Build history of the part. All positions in model axes, mm. A direction names the side the tool comes from. Give positions to 0.01 mm unless a question says otherwise; leave off trailing zeros. Write each loop counter-clockwise with the first axis right and the second up, starting at its lowest first coordinate (ties: lowest second). Pieces come first, ordered by that corner, then holes. Notation, with made-up numbers: (62.25, 54.25) -> (116.25, 54.25) arc R17 ccw to (116.25, 60.25) -> close; hole circle Ø8 at (-25.75, 75). An arc over 180 degrees is marked (long way). One line per question, with ' | ' between items. Start each with the question number.
(1) Tool access for faces 1 (the flat face through (24.25, -5, 59)), 2 (the cylindrical face through (-7.697, -19.028, 89.633)), 3 (the flat face through (8, 17, 91)): list every direction of +Z, -Z, +X, -X, +Y, -Y with a clear straight run to the whole face (end or side of a thin tool).
(2) Band-saw the part on C-C, the plane y = 9. Give the cut face in (x, z).
(3) Drill centre lines: probe 1 along X at (y, z) = (17.8, 91); probe 2 along X at (y, z) = (13.5, 66); probe 3 along Y at (x, z) = (3, 49). Where is each one in solid material? Low to high. Write a range as from..to.
(4) Band-saw the part on B-B, the plane x = -8. Give the cut face in (y, z).
(5) Band-saw the part on A-A, the plane z = 83.5. Give the cut face in (x, y).
(6) Pin check, flat tips, straight feed: P1, Ø8, axis at y = -7, z = 11, coming from the +X side; P2, Ø10, axis at x = 8.5, y = -1.5, coming from the +Z side; P3, Ø4, axis at x = 29, z = 11.5, coming from the -Y side. Stop position of each tip, or through.
(7) Band-saw the part on D-D, the plane z = 11. Give the cut face in (x, y).
(8) Pull direction Z, two halves, no side cores. Call faces 4 (the flat face through (3, 21, 46)), 5 (the flat face through (0, 0, 0)), 6 (the flat face through (23.25, 16, 21)): released by +Z, released by -Z, zero draft, split by the parting line, or undercut.
from build123d import *

# Parameters (mm, degrees)
SKETCH2_W                         = 48.5
SKETCH2_H                         = 42
SKETCH2_W_2                       = 38.5
SKETCH2_H_2                       = 32
SLEEVE_DEPTH                      = 97
SKETCH3_W                         = 48.5
SKETCH3_H                         = 42
REAR_COVER_DEPTH                  = 4
BASKET_CLAMP_DEPTH                = 20
SKETCH5_R                         = 1.4
BASKET_CLAMP_MOUNTING_HOLES_DEPTH = 7
SKETCH7_R                         = 1.4
FRONT_COVER_SCREW_HOLES_TOP_DEPTH = 4
F_1MM_EDGE_FILLETS_R              = 1
BATTERY_INSERTION_CHAMFER_SIZE    = 3
BATTERY_INSERTION_CHAMFER_SIZE2   = 5.196152423


with BuildPart() as part:
    # Sketch2 → Sleeve (new body)
    with BuildSketch(Plane.XY):
        Rectangle(SKETCH2_W, SKETCH2_H)
        Rectangle(SKETCH2_W_2, SKETCH2_H_2, mode=Mode.SUBTRACT)
    extrude(amount=SLEEVE_DEPTH)

    # Sketch3 → Rear Cover (add)
    with BuildSketch(Plane(origin=(0, 0, 0), x_dir=(-1, 0, 0), z_dir=(0, 0, -1))):
        Rectangle(SKETCH3_W, SKETCH3_H)
    extrude(amount=REAR_COVER_DEPTH)

    # Sketch4 → Basket Clamp (add)
    with BuildSketch(Plane(origin=(0, 21, 0), x_dir=(1, 0, 0), z_dir=(0, 1, 0))):
        with BuildLine():
            Line((24.25, 4), (24.25, -36))
            Line((24.25, -36), (30.25, -36))
            Line((30.25, -36), (30.25, -31.5))
            ThreePointArc((30.25, -31.5), (29.047918472, -31.002081528), (28.55, -29.8))
            Line((28.55, -29.8), (28.55, -27.2))
            ThreePointArc((28.55, -27.2), (29.047918472, -25.997918472), (30.25, -25.5))
            Line((30.25, -25.5), (30.25, -6.5))
            ThreePointArc((30.25, -6.5), (29.047918472, -6.002081528), (28.55, -4.8))
            Line((28.55, -4.8), (28.55, -2.2))
            ThreePointArc((28.55, -2.2), (29.047918472, -0.997918472), (30.25, -0.5))
            Line((30.25, -0.5), (30.25, 4))
            Line((30.25, 4), (24.25, 4))
        make_face()
    extrude(amount=-BASKET_CLAMP_DEPTH)

    # Sketch5 → Basket Clamp Mounting Holes (cut)
    with BuildSketch(Plane(origin=(30.25, 0, 0), x_dir=(0, 0, -1), z_dir=(1, 0, 0))):
        with Locations((-21, 16)):
            Circle(SKETCH5_R)
        with Locations((-11, 16)):
            Circle(SKETCH5_R)
        with Locations((-11, 6)):
            Circle(SKETCH5_R)
        with Locations((-21, 6)):
            Circle(SKETCH5_R)
    extrude(amount=-BASKET_CLAMP_MOUNTING_HOLES_DEPTH, mode=Mode.SUBTRACT)

    # Sketch7 → Front Cover Screw Holes Top (cut)
    with BuildSketch(Plane(origin=(0, 21, 0), x_dir=(1, 0, 0), z_dir=(0, 1, 0))):
        with Locations(Location((-8, -91, 0), (0, 0, 180))):
            Circle(SKETCH7_R)
        with Locations(Location((8, -91, 0), (0, 0, 180))):
            Circle(SKETCH7_R)
    front_cover_screw_holes_top = extrude(amount=-FRONT_COVER_SCREW_HOLES_TOP_DEPTH, mode=Mode.SUBTRACT)

    # Front Cover Screw Holes Bottom: Front Cover Screw Holes Top across plane
    add(front_cover_screw_holes_top.mirror(Plane.ZX), mode=Mode.SUBTRACT)

    # 1mm Edge Fillets
    f_1mm_edge_fillets_edges = [part.edges().sort_by_distance(p)[0] for p in [
        (0, -21, -4),
        (-24.25, 0, -4),
        (3, 21, -4),
        (24.25, -10, -4),
        (27.25, 1, -4),
        (24.25, 1, 16),
        (24.25, 11, 36),
        (27.25, 21, 36),
        (-24.25, 21, 46.5),
        (24.25, 21, 66.5),
        (24.25, -21, 46.5),
        (-24.25, -21, 46.5),
    ]]
    fillet(f_1mm_edge_fillets_edges, radius=F_1MM_EDGE_FILLETS_R)

    # Battery Insertion Chamfer
    battery_insertion_chamfer_edges = [part.edges().sort_by_distance(p)[0] for p in [
        (-19.25, 0, 97),
        (0, -16, 97),
        (19.25, 0, 97),
        (0, 16, 97),
    ]]
    battery_insertion_chamfer_side = [part.faces().sort_by_distance(p)[0] for p in [
        (0, 20.358419919, 97),
    ]]
    chamfer(battery_insertion_chamfer_edges, length=BATTERY_INSERTION_CHAMFER_SIZE, length2=BATTERY_INSERTION_CHAMFER_SIZE2, reference=battery_insertion_chamfer_side[0])


solid = part.part
Results:
1) face 1: +Z, +X, -Y | face 2: -Y | face 3: +Y
2) outline: (-24.25, -3) arc R1 ccw to (-23.25, -4) -> (30.25, -4) -> (30.25, 0.5) arc R1.7 cw to (28.55, 2.2) -> (28.55, 4.8) arc R1.7 cw to (30.25, 6.5) -> (30.25, 25.5) arc R1.7 cw to (28.55, 27.2) -> (28.55, 29.8) arc R1.7 cw to (30.25, 31.5) -> (30.25, 36) -> (25.25, 36) arc R1 cw to (24.25, 37) -> (24.25, 97) -> (22.25, 97) -> (19.25, 91.8) -> (19.25, 0) -> (-19.25, 0) -> (-19.25, 91.8) -> (-22.25, 97) -> (-24.25, 97) -> close
3) probe 1: x = -24.25..-9.4, -6.6..6.6, 9.4..24.25 | probe 2: x = -24.25..-19.25, 19.25..24.25 | probe 3: y = -21..-16, 16..21
4) outline: (-21, -3) arc R1 ccw to (-20, -4) -> (20, -4) arc R1 ccw to (21, -3) -> (21, 89.6) -> (17, 89.6) -> (17, 92.4) -> (21, 92.4) -> (21, 97) -> (19, 97) -> (16, 91.8) -> (16, 0) -> (-16, 0) -> (-16, 91.8) -> (-19, 97) -> (-21, 97) -> (-21, 92.4) -> (-17, 92.4) -> (-17, 89.6) -> (-21, 89.6) -> close
5) outline: (-24.25, -20) arc R1 ccw to (-23.25, -21) -> (23.25, -21) arc R1 ccw to (24.25, -20) -> (24.25, 20) arc R1 ccw to (23.25, 21) -> (-23.25, 21) arc R1 ccw to (-24.25, 20) -> close; hole (-19.25, -16) -> (19.25, -16) -> (19.25, 16) -> (-19.25, 16) -> close
6) P1: stops at x = 24.25 | P2: stops at z = 0 | P3: stops at y = 1
7) outline: (-24.25, -20) arc R1 ccw to (-23.25, -21) -> (23.25, -21) arc R1 ccw to (24.25, -20) -> (24.25, 0) arc R1 cw to (25.25, 1) -> (30.25, 1) -> (30.25, 4.6) -> (23.25, 4.6) -> (23.25, 7.4) -> (30.25, 7.4) -> (30.25, 14.6) -> (23.25, 14.6) -> (23.25, 17.4) -> (30.25, 17.4) -> (30.25, 21) -> (-23.25, 21) arc R1 ccw to (-24.25, 20) -> close; hole (-19.25, -16) -> (19.25, -16) -> (19.25, 16) -> (-19.25, 16) -> close
8) face 4: zero draft | face 5: released by +Z | face 6: undercut
